Design review of the part built by this model. Coordinates are the model's own, in mm. A direction names the side the tool comes from. Give positions to 0.01 mm unless a question says otherwise; leave off trailing zeros. Loops run counter-clockwise (first coordinate to the right, second up) from the corner with the lowest first, then second, coordinate; pieces in that order, holes last. Notation, with made-up numbers: (69, -28.5) -> (76, -28.5) arc R6 ccw to (76, -22.5) -> close; hole circle Ø4 at (-4.75, -39). An arc over 180 degrees is marked (long way). Use a Markdown table: item, result. Add a question column.
1. For pin 1 Ø2.5 at (y, z) = (-0.5, 5) entering from -X; pin 2 Ø5.5 at (y, z) = (0, 11) entering from +X; pin 3 Ø5 at (x, z) = (10, -1.5) entering from -Y; pin 4 Ø3 at (x, z) = (14, 19.5) entering from -Y, all flat-tipped, find the tip position at first contact; note any pin that passes through.
2. Add section C-C (z = 12). State the section outline as (x, y) points.
3. For faces 1 (the flat face through (12.5, 0, 7)), 2 (the flat face through (-12.5, 0, 7)), 3 (the flat face through (0, -2.5, 12)), list the 3-axis set-ups (+Z, -Z, +X, -X, +Y, -Y) from which the entire face can be reached by the end or side of a thin tool; tool diameter is ignored.
4. Add section A-A (x = 0). State the section outline as (y, z) points.
5. To check wall thickness, follow line 1 (Y direction, x = -11, z = 2); line 2 (Z direction, x = 4.5, y = -6); line 3 (X direction, y = 8, z = -3). State the ranges of each line that lie inside material, in increasing order.
6. Add section D-D (z = 20.5). State the section outline as (x, y) points, and give its area (3 significant figures).
7. Add section B-B (y = 0). State the section outline as (x, z) points, and give its area (3 significant figures).
Autodesk Inventor part; units mm, degrees
ref_plane "YZ Plane" through (0, 0, 0) normal (1, 0, 0) x (0, 1, 0)
ref_plane "XZ Plane" through (0, 0, 0) normal (0, 1, 0) x (-1, 0, 0)
sketch "Sketch7" plane through (0, 0, 0) normal (0, 1, 0) x (-1, 0, 0)
  line L0 (0, 0) -> (0, 15.7673)
  line L1 (0, 0) -> (-13.3368, 0) construction
  line L2 (0, 15.7673) -> (-13.3368, 0) construction
  line L3 (0, 15.7673) -> (-18.6413, 0) construction
  line L4 (0, 15.7673) -> (-12.4569, -5.231) construction
  line L5 (0, 0) -> (0, -15.7673)
  line L6 (0, -15.7673) -> (-13.3368, 0) construction
  line L7 (0, -15.7673) -> (-18.6413, 0) construction
  line L8 (0, -15.7673) -> (-12.4569, 5.231) construction
  line L9 (-12.4569, 5.231) -> (-18.6413, 0) construction
  line L10 (-9.3537, 0) -> (-18.5948, -7.8164) construction
  line L11 (-9.3537, 0) -> (-18.0926, 7.3915) construction
  line L12 (0, -29.7093) -> (0, 66.7435)
  line L13 (-53.5, -5.9919) -> (-53.5, 6.008)
  line L14 (17.5786, 0) -> (-94.9714, 0)
  line L15 (-15.989, 2.2434) -> (-10.6846, -2.2434) construction
  line L16 (-10.6846, 2.2434) -> (-15.989, -2.2434) construction
  line L17 (-26.151, -15.9303) -> (-40.3783, -15.9303) construction
  line L18 (-40.3783, -15.9303) -> (-40.3783, -12.7539) construction
  line L19 (-40.3783, -12.7539) -> (-26.151, -12.7539) construction
  line L20 (-26.151, -12.7539) -> (-26.151, -15.9303) construction
  point P0 (-53.5, 0)
  dimension "Roller_Side_difference" = -0.0003
  dimension "d90" = 15.7673
  dimension "d201" = 53.5
  dimension "d343" = 99.548
  dimension "d344" = 99.549
  dimension "d367" = 8.1
sketch "Sketch1" plane through (0, 0, 0) normal (0, 0, 1) x (1, 0, 0)
  circle A0 centre (0, 0) radius 13.3368 construction
  line L0 (0, 0) -> (13.3368, 0)
  line L1 (0, 0) -> (13.3368, 4.025)
  line L2 (13.3368, 0) -> (13.3368, 4.025)
  circle A1 centre (0, 0) radius 53.5
  point P0 (56.8, 0)
  dimension "d56" = 13.3368
  dimension "d57" = 4.025
  dimension "d400" = 53.5
  dimension "d495" = 2.5
  dimension "d496" = 8
  dimension "d531" = 5.5
  dimension "d532" = 5.5
  dimension "d533" = 5.5
  dimension "d537" = 24.5
  dimension "d538" = 3
  dimension "d543" = 5.5
  dimension "d549" = 3
  dimension "d550" = 3
  dimension "d567" = 5.5
  dimension "d568" = 5.5
sketch "Roller1" plane through (0, 0, 0) normal (0, 1, 0) x (-1, 0, 0)
  line L0 (0, 15.7673) -> (-12.4569, -5.231) construction
  line L1 (0, 15.7673) -> (-18.6413, 0) construction
  line L2 (-9.3537, 0) -> (-18.0926, 7.3915) construction
  line L3 (0, -15.7673) -> (-18.6413, 0) construction
  line L4 (-9.4248, -0.0708) -> (-12.4245, -5.1274)
  line L5 (-12.4245, -5.1274) -> (-18.5445, 0.0491)
  line L6 (-18.5445, 0.0491) -> (-14.0556, 3.846)
  line L7 (-14.0556, 3.846) -> (-9.4248, -0.0708)
  line L8 (-11.7456, 1.8921) -> (-15.4898, -2.5346)
  line L9 (-10.9821, 1.2463) -> (-14.7263, -3.1804)
  point P0 (0, 0)
  point P1 (-15.4845, -2.5391)
  dimension "d345" = 0.025
  dimension "d346" = 0.025
  dimension "d347" = 0.1
  dimension "d348" = 0.1
  dimension "d349" = 99.549
  dimension "d350" = 99.548
  dimension "d357" = 1
  dimension "d369" = 4.0148
sketch "Roller2" plane through (0, 0, 0) normal (0, 1, 0) x (-1, 0, 0)
  line L0 (0, -15.7673) -> (-12.4569, 5.231) construction
  line L1 (-9.3537, 0) -> (-18.5948, -7.8164) construction
  line L2 (0, -15.7673) -> (-18.6413, 0) construction
  line L3 (0, 15.7673) -> (-18.6413, 0) construction
  line L4 (-12.4245, 5.1274) -> (-9.4248, 0.0708)
  line L5 (-9.4248, 0.0708) -> (-14.0556, -3.846)
  line L6 (-14.0556, -3.846) -> (-18.5445, -0.0491)
  line L7 (-18.5445, -0.0491) -> (-12.4245, 5.1274)
  line L8 (-15.4845, 2.5391) -> (-11.7403, -1.8876)
  line L9 (-14.721, 3.1849) -> (-10.9767, -1.2418)
  point P0 (0, 0)
  dimension "d351" = 0.025
  dimension "d352" = 0.025
  dimension "d354" = 0.1
  dimension "d355" = 99.548
  dimension "d356" = 99.549
  dimension "d370" = 0.1
  dimension "d371" = 1
sketch "Sketch22" plane through (0, 0, 0) normal (0, 1, 0) x (-1, 0, 0)
  line L0 (-31.756, 8.0215) -> (-17.5287, 8.0215) construction
  line L1 (-17.5287, 8.0215) -> (-17.5287, 4.8451) construction
  line L2 (-17.5287, 4.8451) -> (-31.756, 4.8451) construction
  line L3 (-31.756, 4.8451) -> (-31.756, 8.0215) construction
  point P0 (0, 0)
  dimension "Roller_Side_difference" = -0.0003
sketch "Sketch2" plane through (0, 0, 0) normal (0, 1, 0) x (-1, 0, 0)
  line L0 (0, 0) -> (0, 13.3368) construction
  line L1 (0, 0) -> (-13.3368, 0)
  line L2 (0, 0) -> (0, -13.3368)
  line L3 (0, -13.3368) -> (-13.3368, 0) construction
  line L4 (0, 13.3368) -> (-13.3368, 0) construction
  line L5 (-78.8928, 52.9645) -> (0, 13.3368) construction
  line L6 (-34.8011, 15.91) -> (0, 13.3368) construction
  line L7 (-34.8011, 15.91) -> (0, -13.3368) construction
  line L8 (-48.3339, 16.9106) -> (0, -13.3368) construction
  point P0 (-17.4708, -4.134)
sketch "Sketch23" plane through (0, 0, 0) normal (0, 1, 0) x (-1, 0, 0)
  line L0 (0, -15.7673) -> (-12.4569, 5.231) construction
  line L1 (0, -15.7673) -> (-18.6413, 0) construction
  line L2 (0, 15.7673) -> (-12.4569, -5.231) construction
  line L3 (-12.4569, 5.231) -> (-18.6413, 0) construction
  line L4 (0, 15.7673) -> (-18.6413, 0) construction
  line L5 (-12.4569, 5.231) -> (-12.4569, -5.231) construction
  line L6 (17.5786, 0) -> (-94.9714, 0)
  line L7 (-11.4508, 3.731) -> (-9.2677, 0.051)
  line L8 (-9.2677, -0.051) -> (-11.4508, -3.731)
  line L9 (-14.3852, 3.731) -> (-18.7059, 0.0764)
  line L10 (-18.7059, -0.0764) -> (-14.3852, -3.731)
  arc A0 (-18.7059, 0.0764) -> (-18.7059, -0.0764) centre (-18.6413, 0) ccw
  arc A1 (-9.2677, -0.051) -> (-9.2677, 0.051) centre (-9.3537, 0) ccw
  line L11 (-11.4508, 3.731) -> (-11.4508, 5.231)
  line L12 (-11.4508, 5.231) -> (-1, 5.231)
  line L13 (-1, 5.231) -> (-1, -5.231)
  line L14 (-1, -5.231) -> (-11.4508, -5.231)
  line L15 (-11.4508, -5.231) -> (-11.4508, -3.731)
  line L16 (-14.3852, 3.731) -> (-14.3852, 5.231)
  line L17 (-14.3852, 5.231) -> (-53.5, 5.231)
  line L18 (-53.5, 5.231) -> (-53.5, -5.231)
  line L19 (-14.3852, -3.731) -> (-14.3852, -5.231)
  line L20 (-14.3852, -5.231) -> (-53.5, -5.231)
  line L21 (-12.4569, 5.231) -> (-12.4569, 5.231)
  line L22 (-12.4569, -5.231) -> (-12.4569, -5.231)
  line L23 (0, -29.7093) -> (0, 66.7435)
  line L24 (-18.7962, 0) -> (-53.5, 0)
  point P0 (0, 0)
  point P1 (-9.2374, 0)
  point P2 (-18.7413, 0)
  point P3 (-53.5, 0)
  dimension "d378" = 90
  dimension "d379" = 0.1
  dimension "d380" = 0.1
  dimension "d381" = 0.1
  dimension "d382" = 0.1
  dimension "d383" = 0.1
  dimension "d384" = 10.4619
  dimension "d385" = 0
  dimension "d386" = 0
  dimension "d391" = 1
  dimension "d392" = 53.5
  dimension "d393" = 1.5
  dimension "d394" = 1.5
  dimension "d395" = 1.5
  dimension "d396" = 1.5
sketch "Sketch44" plane through (0, 0, 0) normal (0, 1, 0) x (-1, 0, 0)
  line L0 (-18.7962, 0) -> (3.1509, -18.5634)
  line L1 (17.5786, 0) -> (-94.9714, 0)
  line L2 (-11.4508, 5.231) -> (-1, 5.231)
  line L3 (-14.3852, 5.231) -> (-53.5, 5.231)
  line L4 (0, 0) -> (0, 15.7673)
  line L5 (0, 0) -> (0, -15.8983)
  line L6 (-25.707, -7.6404) -> (3.3976, -7.6404)
  line L7 (-18.6413, 0) -> (0, -15.7673)
  point P0 (-3.6044, 0)
  point P1 (-9.6083, -7.6404)
  point P2 (0, -7.6404)
  dimension "d615" = 0.1
revolve "Revolution17" add sketch "Sketch44" angle 360 about axis through (0, 0, 0) along (0, 0, 1) contours L1 L5 L6 L7
sketch "Sketch45" plane through (0, 0, 0) normal (0, 0, 1) x (1, 0, 0)
  line L0 (-12.5, 2.5) -> (12.5, 2.5)
  line L1 (12.5, 2.5) -> (12.5, -2.5)
  line L2 (12.5, -2.5) -> (-12.5, -2.5)
  line L3 (-12.5, -2.5) -> (-12.5, 2.5)
  line L4 (-12.5, 2.5) -> (12.5, -2.5) construction
  line L5 (12.5, 2.5) -> (-12.5, -2.5) construction
  point P0 (0, 0)
  dimension "d617" = 25
  dimension "d618" = 5
extrude "Extrusion39" add sketch "Sketch45" along normal blind 25
fillet "Fillet4" radius 10 2 edges at (-12.5, 0, 25) (12.5, 0, 25)
fillet "Fillet5" radius 0.5 1 edges at (-18.6413, 0, 0)
sketch "Sketch40" plane through (0, 0, -5.231) normal (0, 0, -1) x (-1, 0, 0)
  circle A0 centre (53.5, 0) radius 2.75
  circle A1 centre (0, 0) radius 53.5
  point P0 (53.4293, 2.7491)
  point P1 (53.4293, -2.7491)
  dimension "d585" = 8
  dimension "d587" = 1.75
  dimension "d589" = 3
  dimension "d592" = 2
  dimension "d593" = 12
  dimension "d594" = 12
  dimension "d611" = 360
equation "\"Roller_Side_difference\" = -0.001568deg"
equation "\"Cycloid_Top_Plate_Fasner_Inner\" = 61.25"
equation "\"Cycloid_Top_Plate_Fasner_Outer\" = 85.75"
equation "\"Roller_Hole_Radius\" = 1"
equation "\"Distance_To_Bearing\" = 20.65135"
equation "\"d514\" = 0.2"
properties part number "OuterRaceTool"
Taken from the geometry:
| question | item | result |
|---|---|---|
| 1 | pin 1 | stops at x = -12.5 |
| 1 | pin 2 | stops at x = 12.5 |
| 1 | pin 3 | stops at y = -16.03 |
| 1 | pin 4 | passes through |
| 2 | outline | (-12.5, -2.5) -> (12.5, -2.5) -> (12.5, 2.5) -> (-12.5, 2.5) -> close |
| 3 | face 1 | +Z, +X, +Y, -Y |
| 3 | face 2 | +Z, -X, +Y, -Y |
| 3 | face 3 | +Z, +X, -X, -Y |
| 4 | outline | (-17.6, -0.88) -> (-9.61, -7.64) -> (9.61, -7.64) -> (17.6, -0.88) arc R0.5 ccw to (17.28, 0) -> (2.5, 0) -> (2.5, 25) -> (-2.5, 25) -> (-2.5, 0) -> (-17.28, 0) arc R0.5 ccw to start |
| 5 | line 1 | y = -2.5 to 2.5 |
| 5 | line 2 | z = -7.64 to 0 |
| 5 | line 3 | x = -12.8 to 12.8 |
| 6 | outline | (-10.85, -2.5) -> (10.85, -2.5) -> (10.85, 2.5) -> (-10.85, 2.5) -> close |
| 6 | area | 109 mm^2 |
| 7 | outline | (-17.6, -0.88) -> (-9.61, -7.64) -> (9.61, -7.64) -> (17.6, -0.88) arc R0.5 ccw to (17.28, 0) -> (12.5, 0) -> (12.5, 15) arc R10 ccw to (2.5, 25) -> (-2.5, 25) arc R10 ccw to (-12.5, 15) -> (-12.5, 0) -> (-17.28, 0) arc R0.5 ccw to start |
| 7 | area | 797 mm^2 |
